```python
from build123d import *

# Parameters (mm, degrees)
F1_DEPTH = 7
F2_T     = -3
F3_DEPTH = 25


with BuildPart() as f1:
    # F0 (on Top) → F1 (new body)
    with BuildSketch(Plane.XY):
        Polygon((-32.5, 18), (-17.5, 0), (-17.5, -38), (-57.5, -38), (-75.5, -23), (-75.5, -88), (-57.5, -73), (-17.5, -73), (-17.5, -144), (-32.5, -162), (32.5, -162), (17.5, -144), (17.5, -73), (57.5, -73), (75.5, -88), (75.5, -23), (57.5, -38), (17.5, -38), (17.5, 0), (32.5, 18), align=None)
    extrude(amount=F1_DEPTH)

    # F2
    f2_openings = [f1.faces().sort_by_distance(p)[0] for p in [
        (0, -65.365385, 7),
    ]]
    offset(amount=F2_T, openings=f2_openings, kind=Kind.INTERSECTION)

    # F3 (cut): a face of the model
    f3_faces = [f1.faces().sort_by_distance(p)[0] for p in [
        (0, -65.2824145306, 3),
    ]]
    extrude(f3_faces, amount=-F3_DEPTH, mode=Mode.SUBTRACT)


solid = f1.part
```
Here's how the part is built. I have some questions about the finished solid (model axes, mm). A direction names the side the tool comes from. Round coordinates to 2 decimals unless told otherwise and drop trailing zeros. Order: outer loops, then holes, each group sorted by start corner. A loop starts at its lowest first (then second) coordinate and runs counter-clockwise, first axis right, second up. Notation, with made-up numbers: (78, 66.25) -> (98, 66.25) arc R20 ccw to (98, 88.25) -> close; hole circle Ø2 at (30, 27). An arc over 180 degrees is marked (long way). Use a Markdown table: item, result. Add a question column.
(1) For pin 1 Ø1.5 at (x, z) = (53, 3) entering from +Y; pin 2 Ø3.5 at (y, z) = (-14, 3.5) entering from +X; pin 3 Ø2 at (y, z) = (-20, 2) entering from -X, each with a flat end and sliding along its axis, tell me the tip position at first contact or that it passes through.
(2) Suppose I cut it at A-A, the plane y = -102. Please give me the cut outline in (x, z).
(3) I need wall thicknesses on line 1 along Y through (x, z) = (-55, 5); line 2 along X through (y, z) = (-11, 3.75); line 3 along Y through (x, z) = (-20, 3.75). Which ranges of each line are inside material? Lowest first, please.
(4) Suppose I cut it at D-D, the plane y = -25. Please give me the cut outline in (x, z), and give its area (3 significant figures).
(5) Suppose I cut it at B-B, the plane x = 34.5. Please give me the cut outline in (y, z), and give its area (3 significant figures).
(6) For faces 5 (the face through (-25, 9, 3)), 6 (the face through (-66.626, -80.605, 3.451)), 7 (the face through (0, -159, 4)), which set-ups out of +Z, -Z, +X, -X, +Y, -Y let a thin tool reach every point of the face, with its end or its side?
(7) Suppose I cut it at C-C, the plane x = -30.5. Please give me the cut outline in (y, z), and give its area (3 significant figures).
(8) If we mould it in two halves opening along X, with no side actions, what happens to faces 1 (the face through (-17, -72, 7)), 2 (the face through (-25, -153, 3)), 3 (the face through (25, -153, 3)), 4 (the face through (-65.64, -75.88, 3.55))? For each: released by +X, released by -X, zero draft, split by the parting line, or undercut.
Verdict:
| question | item | result |
|---|---|---|
| 1 | pin 1 | y = -38 |
| 1 | pin 2 | x = 17.5 |
| 1 | pin 3 | x = -17.5 |
| 2 | outline | (-17.5, 0) -> (-14.5, 0) -> (-14.5, 7) -> (-17.5, 7) -> close; (14.5, 0) -> (17.5, 0) -> (17.5, 7) -> (14.5, 7) -> close |
| 3 | line 1 | -73 to -70, -41 to -38 |
| 3 | line 2 | -17.5 to -14.5, 14.5 to 17.5 |
| 3 | line 3 | -162 to -159, -151.69 to -147, -73 to -70, -41 to -38, 3 to 7.69, 15 to 18 |
| 4 | outline | (-75.5, 0) -> (-73.1, 0) -> (-73.1, 7) -> (-75.5, 7) -> close; (-17.5, 0) -> (-14.5, 0) -> (-14.5, 7) -> (-17.5, 7) -> close; (14.5, 0) -> (17.5, 0) -> (17.5, 7) -> (14.5, 7) -> close; (73.1, 0) -> (75.5, 0) -> (75.5, 7) -> (73.1, 7) -> close |
| 4 | area | 75.6 mm2 |
| 5 | outline | (-73, 0) -> (-70, 0) -> (-70, 7) -> (-73, 7) -> close; (-41, 0) -> (-38, 0) -> (-38, 7) -> (-41, 7) -> close |
| 5 | area | 42.0 mm2 |
| 6 | face 5 | +Z, -Z, -X |
| 6 | face 6 | +Z, -Z, -Y |
| 6 | face 7 | +Z, -Z |
| 7 | outline | (-162, 0) -> (-159.6, 0) -> (-159.6, 7) -> (-162, 7) -> close; (-73, 0) -> (-70, 0) -> (-70, 7) -> (-73, 7) -> close; (-41, 0) -> (-38, 0) -> (-38, 7) -> (-41, 7) -> close; (15.6, 0) -> (18, 0) -> (18, 7) -> (15.6, 7) -> close |
| 7 | area | 75.6 mm2 |
| 8 | face 1 | zero draft |
| 8 | face 2 | released by -X |
| 8 | face 3 | released by +X |
| 8 | face 4 | undercut |
